Read the model definition and answer for the solid it produces. Units are mm, in the model's axes. Face numbers are marked on the shaded views. A direction names the side the tool comes from. Round coordinates to 2 decimals unless told otherwise and drop trailing zeros. Order: outer loops, then holes, each group sorted by start corner. A loop starts at its lowest first (then second) coordinate and runs counter-clockwise, first axis right, second up. Notation, with made-up numbers: (-1.75, 5.5) - (20.25, 5.5) arc R14 cw to (20.25, 10.5) - close; hole circle Ø10 at (12.5, -12.75). An arc over 180 degrees is marked (long way). Put each result on its own line as item: value. Start each with the question number.
Q1. For a pull along Z with two mould halves and no side action, classify the marked faces 1, 2 and 3 as pulls with the +Z half, pulls with the -Z half, needs draft (parallel to the pull), parting line crosses it, or undercut.
Q2. Section B-B on z = 3 is taken. Give the vertices of the cut face in (x, y).
Q3. Each of these flat-tipped pins is pushed along its axis until it touches: pin 1 Ø2 at (y, z) = (1.5, 2) entering from +X; pin 2 Ø0.6 at (x, z) = (1.5, 10.5) entering from -Y; pin 3 Ø0.6 at (x, z) = (1, 10.5) entering from +Y; pin 4 Ø1 at (x, z) = (-2, 3) entering from -Y. Where does it stop, or does it pass through?
Q4. Which of the six approach directions +Z, -Z, +X, -X, +Y, -Y give full straight-line access (tool end or side, diameter ignored) to the marked faces 4, 5 and 6?
Q5. Find the intervals of material crossed by line 1 along Y through (x, z) = (0.8, 9.25); line 2 along Y through (x, z) = (1.7, 9.75); line 3 along Z through (x, y) = (0.35, 1.95), in increasing order. Write a range as from..to.
Autodesk Inventor part; units mm, degrees
ref_plane "Work Plane1" through (0, 0, 4.5) normal (0, 0, 1) x (1, 0, 0)
ref_plane "Work Plane3" through (-4.9804, 0, 1.8127) normal (0.9396926, 0, -0.3420201) x (0, 1, 0)
ref_plane "Work Plane4" through (0, 3, 0) normal (0, 1, 0) x (-1, 0, 0)
sketch "Sketch1" plane through (0, 0, 0) normal (0, 0, 1) x (1, 0, 0)
  circle A0 centre (0, 0) radius 1.1
  dimension "d0" = 2.2
extrude "Extrusion1" add sketch "Sketch1" along normal blind 5.6
ref_plane "Work Plane1" through (0, 0, 4.5) normal (0, 0, 1) x (1, 0, 0)
sketch "Sketch2" plane through (0, 0, 4.5) normal (0, 0, 1) x (1, 0, 0)
  circle A0 centre (0, 0) radius 1.1
  circle A1 centre (0, 0) radius 1.2
  dimension "d4" = 0.1
extrude "Extrusion2" add sketch "Sketch2" against normal blind 0.2
chamfer "Chamfer1" distance 0.1 angle 45 1 edges at (-1.2, 0, 4.3)
fillet "Fillet1" radius 0.2 1 edges at (-1.1, 0, 0)
sketch "Sketch3" plane through (0, 0, 5.6) normal (0, 0, 1) x (1, 0, 0)
  circle A0 centre (0, 0) radius 1.1
  circle A1 centre (0, 0) radius 1.3
  dimension "d11" = 0.2
extrude "Extrusion3" add sketch "Sketch3" along normal blind 3 contours A0 | A1
ref_plane "Work Plane3" through (-4.9804, 0, 1.8127) normal (0.9396926, 0, -0.3420201) x (0, 1, 0)
ref_plane "Work Plane2" through (0, 0, 0) normal (0.9396926, 0, -0.3420201) x (0, 1, 0)
sketch "Sketch4" plane through (-4.9804, 0, 1.8127) normal (0.9396926, 0, -0.3420201) x (0, 1, 0)
  ellipse E0 centre (0, 5.2623) end of major axis (1.3, 5.2623) minor radius 0.4446
  line L0 (-1.3, 5.2623) -> (-1.3, 8.0814)
  circle A0 centre (0, 8.8623) radius 2.45
  point P0 (0, 0)
  dimension "d16" = 4.9
  dimension "d17" = 3.6
  dimension "d18" = 1.3
extrude "Extrusion4" add sketch "Sketch4" along normal blind 4.5 contours A0
sketch "Sketch5" plane through (-1.9493, 0, 10.1405) normal (-0.9396926, 0, 0.3420201) x (0.3420201, 0, 0.9396926)
  circle A0 centre (0, 0) radius 2.45
  arc A1 (0.6652, 1.4) -> (0.6652, -1.4) centre (0, 0) ccw
  line L0 (0.6652, 1.4) -> (3.89, 1.4)
  line L1 (3.89, 1.4) -> (3.89, -1.4)
  line L2 (3.89, -1.4) -> (0.6652, -1.4)
  point P0 (-8.8623, 0)
  dimension "d21" = 0.9
  dimension "d22" = 1.4
  dimension "d23" = 1.4
  dimension "d25" = 3.89
extrude "Extrusion5" cut sketch "Sketch5" against normal blind 4.5 contours A0 L2 A1 L0 | A0 L0 L1 L2 picked at (1.2601, 0)
ref_plane "Work Plane4" through (0, 3, 0) normal (0, 1, 0) x (-1, 0, 0)
sketch "Sketch6" plane through (0, 3, 0) normal (0, 1, 0) x (-1, 0, 0)
  line L0 (-1.0876, 11.1748) -> (1.2616, 12.0299)
  line L1 (2.0243, 9.9344) -> (1.2616, 12.0299)
  arc A0 (2.0243, 9.9344) -> (-1.0876, 11.1748) centre (-0.227, 8.8102) ccw
  point P0 (0, 0)
  dimension "d29" = 2.5
  dimension "d30" = 2.23
extrude "Extrusion6" cut sketch "Sketch6" against normal through all
properties part number "Lego hand"
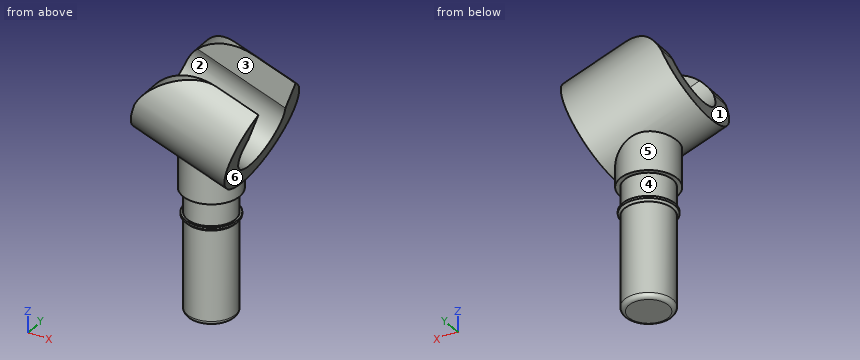
Findings:
1. face 1: pulls with the +Z half
1. face 2: undercut
1. face 3: needs draft
2. outline: circle Ø2.2 at (0, 0)
3. pin 1: x = 0.98
3. pin 2: y = -2.13
3. pin 3: y = 2.22
3. pin 4: through
4. face 4: none
4. face 5: -Z
4. face 6: -Z, +X, +Y, -Y
5. line 1: -2.45..-1.55, 1.55..2.45
5. line 2: -2.29..-1.4, 1.4..2.29
5. line 3: 7.73..10.88
